For this review, take the finished solid that the model builds, in its own axes (mm). A direction names the side the tool comes from. Round coordinates to 2 decimals unless told otherwise and drop trailing zeros. Loops run counter-clockwise (first coordinate to the right, second up) from the corner with the lowest first, then second, coordinate; pieces in that order, holes last. Notation, with made-up numbers: M 5,-37 L 20,-37 A15 ccw 20,-22 Z; hole C 17,52.5 d10. An arc over 180 degrees is marked long. One line per question, with ' | ' between items. Start each with the question number.
1) For faces 1 (the face through (-6, 2.778, -39)), 2 (the face through (0.1, 3.1, -12.7)), list the 3-axis set-ups (+Z, -Z, +X, -X, +Y, -Y) from which the entire face can be reached by the end or side of a thin tool; tool diameter is ignored.
2) We need section B-B (y = 1). State how many separate pieces and enclosed holes the cut face has, and give its area (3 significant figures).
3) We need section A-A (z = -17). Give the boundary of the cut face in (x, y).
4) For pin 1 Ø5 at (x, z) = (0, 9.525) entering from -Y, flat-tipped, find the tip position at first contact; note if it passes through.
5) Mouldability with a two-part tool opening along Z and no side actions: class faces 3 (the face through (-9.078, 3.19, 43.806)), 4 (the face through (0.42, 4.59, -44.44)), 5 (the face through (-12.7, 3, 0)), 6 (the face through (8.881, 3.19, -44.003)) as pulls with the +Z half, pulls with the -Z half, needs draft (parallel to the pull), parting line crosses it, or undercut.
6) We need section D-D (z = -27). Give the boundary of the cut face in (x, y), and give its area (3 significant figures).
7) For probe 1 along Z at (x, y) = (-0.25, 2.5); probe 2 along X at (y, z) = (2.5, 9); probe 3 along Z at (x, y) = (-3.75, 2.5), list the stretches that pass through material, from the lowest coordinate up. Write a range as from..to.
```python
from build123d import *

# Parameters (mm, degrees)
SKETCH1_W           = 25.4
SKETCH1_H           = 95.25
SKETCH1_R           = 3.175
BOSS_EXTRUDE1_DEPTH = 6.35
FILLET1_R           = 12.7
FILLET2_R           = 2.116666667
SKETCH5_R           = 9.525
SKETCH5_R_2         = 7.016807895
CUT_EXTRUDE2_DEPTH  = 3.571875
SKETCH5_2_R         = 7.016807895
CUT_EXTRUDE3_DEPTH  = 6.35


with BuildPart() as part:
    # Sketch1 → Boss-Extrude1 (new body)
    with BuildSketch(Plane(origin=(0, 0, 0), x_dir=(1, 0, 0), z_dir=(0, 1, 0))):
        Rectangle(SKETCH1_W, SKETCH1_H)
        with Locations(Location((0, 9.525, 0), (0, 0, 270))):
            Circle(SKETCH1_R, mode=Mode.SUBTRACT)
        with Locations(Location((0, -9.525, 0), (0, 0, 270))):
            Circle(SKETCH1_R, mode=Mode.SUBTRACT)
    extrude(amount=BOSS_EXTRUDE1_DEPTH)

    # Fillet1
    fillet1_edges = [part.edges().sort_by_distance(p)[0] for p in [
        (-12.7, 3.175, -47.625),
        (12.7, 3.175, -47.625),
        (-12.7, 3.175, 47.625),
        (12.7, 3.175, 47.625),
    ]]
    fillet(fillet1_edges, radius=FILLET1_R - 0.0001)  # a hair under: the kernel refuses the full size

    # Fillet2
    fillet2_edges = [part.edges().sort_by_distance(p)[0] for p in [
        (-12.7, 0, 0),
        (-12.7, 6.35, 0),
        (12.7, 0, 0),
        (8.98028541, 0, 43.90528541),
        (-8.98028541, 0, 43.90528541),
        (8.98028541, 0, -43.90528541),
        (-8.98028541, 0, -43.90528541),
        (12.7, 6.35, 0),
        (8.98028541, 6.35, 43.90528541),
        (-8.98028541, 6.35, 43.90528541),
        (8.98028541, 6.35, -43.90528541),
        (-8.98028541, 6.35, -43.90528541),
    ]]
    fillet(fillet2_edges, radius=FILLET2_R)

    # Sketch5 → Cut-Extrude2 (cut)
    with BuildSketch(Plane(origin=(0, 6.35, 0), x_dir=(1, 0, 0), z_dir=(0, 1, 0))):
        with Locations(Location((0, 34.925, 0), (0, 0, 270))):
            Circle(SKETCH5_R)
        with Locations(Location((0, 34.925, 0), (0, 0, 270))):
            Circle(SKETCH5_R_2, mode=Mode.SUBTRACT)
    extrude(amount=-CUT_EXTRUDE2_DEPTH, mode=Mode.SUBTRACT)

    # Sketch5<2> → Cut-Extrude3 (cut)
    with BuildSketch(Plane(origin=(0, 6.35, 0), x_dir=(1, 0, 0), z_dir=(0, 1, 0))):
        with Locations(Location((0, 34.925, 0), (0, 0, 270))):
            Circle(SKETCH5_2_R)
    extrude(amount=-CUT_EXTRUDE3_DEPTH, mode=Mode.SUBTRACT)


solid = part.part
```
Answers below:
1) face 1: +Y | face 2: +Y, -Y
2) separate pieces: 1 | enclosed holes: 3 | area: 1,990 mm^2
3) outline: M -12.7,2.12 A2.12 ccw -10.58,0 L 10.58,0 A2.12 ccw 12.7,2.12 L 12.7,4.23 A2.12 ccw 10.58,6.35 L -10.58,6.35 A2.12 ccw -12.7,4.23 Z
4) pin 1: through
5) face 3: pulls with the +Z half | face 4: undercut | face 5: needs draft | face 6: pulls with the -Z half
6) outline: M -12.7,2.12 A2.12 ccw -10.58,0 L 10.58,0 A2.12 ccw 12.7,2.12 L 12.7,4.23 A2.12 ccw 10.58,6.35 L 5.28,6.35 L 5.28,2.78 L -5.28,2.78 L -5.28,6.35 L -10.58,6.35 A2.12 ccw -12.7,4.23 Z | area: 120 mm^2
7) probe 1: -47.62..-41.94, -27.91..-12.69, -6.36..6.36, 12.69..47.62 | probe 2: -12.7..-3.13, 3.13..12.7 | probe 3: -47.06..-40.86, -28.99..47.06
